Source: CAD feature listing. Evaluate the final solid. Frame: model axes, mm. Face numbers are marked on the shaded views. A direction names the side the tool comes from. Give positions to 0.01 mm unless a question says otherwise; leave off trailing zeros. Write each loop counter-clockwise with the first axis right and the second up, starting at its lowest first coordinate (ties: lowest second). Pieces come first, ordered by that corner, then holes. Notation, with made-up numbers: (56, 59.25) -> (101, 59.25) arc R27 cw to (101, 79.25) -> close; hole circle Ø3 at (85, 56.25). An arc over 180 degrees is marked (long way). Use one line per item in the form item = value. Start each with the question number.
(1) Draft query along X for the marked faces 1, 2 and 3. Return one class per face: pulls with the +X half, pulls with the -X half, needs draft (parallel to the pull), parting line crosses it, or undercut.
(2) First-contact query: P1, Ø2.5, axis at x = 47, y = 22.5, coming from the -Z side; P2, Ø12, axis at x = 46.5, z = 16.5, coming from the +Y side; P3, Ø6.5, axis at y = 37, z = 72, coming from the -X side. Flat tips, straight axial feed; report the tip coordinate or a pass-through.
(3) Material intervals for line 1 along Y through (x, z) = (45.6, 72.9); line 2 along Y through (x, z) = (48.9, 72.9); line 3 along X through (y, z) = (25.5, 75.5), sorted ascending. Write a range as from..to.
(4) Cut plane B-B, the plane y = 32. Output: boundary loops of the cut face in (x, z).
(5) Set-up query: the marked faces 4, 5 and 6. Return all of +Z, -Z, +X, -X, +Y, -Y with unobstructed straight access to the full face (end or side cutting, diameter ignored); none if empty.
(6) Cut plane A-A, the plane z = 56. Output: boundary loops of the cut face in (x, y).
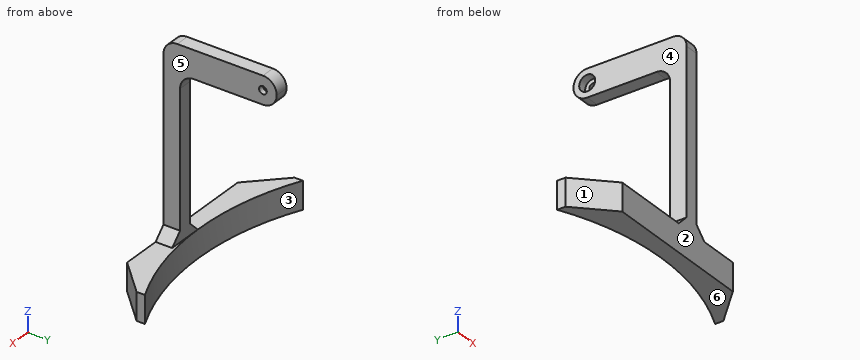
Autodesk Inventor part; units mm, degrees
ref_plane "YZ Plane" through (0, 0, 0) normal (1, 0, 0) x (0, 1, 0)
ref_plane "XZ Plane" through (0, 0, 0) normal (0, 1, 0) x (-1, 0, 0)
ref_plane "XY Plane" through (0, 0, 0) normal (0, 0, 1) x (1, 0, 0)
sketch "Esquisse1" plane through (0, 0, 0) normal (0, 0, 1) x (1, 0, 0)
  line L0 (0, 0) -> (0, 15)
  line L1 (0, 0) -> (80, 0)
  line L2 (80, 0) -> (80, 15)
  arc A0 (0, 15) -> (80, 15) centre (40, 99.3889) ccw
  line L3 (0, 6) -> (80, 6) construction
  line L4 (40, 0) -> (40, 6) construction
  dimension "d0" = 15
  dimension "d1" = 80
  dimension "d28" = 6
extrude "Extrusion1" add sketch "Esquisse1" along normal blind 10
sketch "Esquisse2" plane through (0, 0, 10) normal (0, 0, 1) x (1, 0, 0)
  line L0 (0, 0) -> (80, 0)
  line L1 (44.6, 0) -> (49.6, 0)
  line L2 (49.6, 0) -> (49.6, 6)
  line L3 (49.6, 6) -> (44.6, 6)
  line L4 (44.6, 6) -> (44.6, 0)
  line L5 (0, 15) -> (0, 0)
  line L6 (0, 6) -> (80, 6) construction
  line L7 (80, 0) -> (80, 15)
  arc A0 (0, 15) -> (80, 15) centre (40, 99.3889) ccw
  line L8 (40, 0) -> (40, 6) construction
  dimension "d6" = 5
  dimension "d9" = 80
  dimension "d11" = 6
  dimension "d27" = 4.6
extrude "Extrusion2" add sketch "Esquisse2" along normal blind 67.9 contours L4 L3 L2 L0
sketch "Esquisse6" plane through (44.6, 6, 10) normal (0, 1, 0) x (1, 0, 0)
  line L0 (5, 0) -> (5, -67.9)
  line L1 (0, 0) -> (0, -67.9)
  line L2 (5, -67.9) -> (0, -67.9)
  line L3 (0, -67.9) -> (0, -57.9)
  line L4 (0, -57.9) -> (5, -57.9)
  line L5 (5, -57.9) -> (5, -67.9)
  point P0 (-44.6, 10)
  point P1 (5, -57.9)
  dimension "d29" = 10
extrude "Extrusion5" add sketch "Esquisse6" along normal blind 35
sketch "Esquisse7" plane through (44.6, 0, 10) normal (-1, 0, 0) x (0, 0, 1)
  line L0 (67.9, 41) -> (57.9, 41) construction
  line L1 (62.9, 41) -> (62.9, 0) construction
  line L2 (0, 0) -> (67.9, 0) construction
  circle A0 centre (62.9, 36) radius 2.9
  circle A1 centre (62.9, 36) radius 1.4
  point P0 (-10, 0)
  dimension "d38" = 2.8
  dimension "d53" = 5.8
  dimension "d54" = 5
extrude "Extrusion6" cut sketch "Esquisse7" against normal up to surface (5 mm away) contours A1
chamfer "Chanfrein1" distance 4 angle 45 2 edges at (44.6, 3, 10) (49.6, 3, 10)
fillet "Congé1" radius 5 2 edges at (47.1, 0, 77.9) (47.1, 6, 67.9)
fillet "Congé2" radius 5 2 edges at (47.1, 41, 77.9) (47.1, 41, 67.9)
chamfer "Chanfrein2" distance 12 angle 45 2 edges at (0, 0, 5) (80, 0, 5)
extrude "Extrusion8" cut sketch "Esquisse7" against normal blind 3
properties part number "_Impression 3D"
Geometry says:
q1.face_1 = pulls with the -X half
q1.face_2 = needs draft
q1.face_3 = undercut
q2.P1 = 67.9
q2.P2 = 6
q2.P3 = 44.6
q3.line_1 = 0..33.1, 38.9..41
q3.line_2 = 0..34.6, 37.4..41
q3.line_3 = 44.6..49.6
q4.outline = (44.6, 67.9) -> (49.6, 67.9) -> (49.6, 77.9) -> (44.6, 77.9) -> close
q5.face_4 = +Z, -X, +Y, -Y
q5.face_5 = +Z, +X, +Y, -Y
q5.face_6 = -Z, +X, -X, +Y, -Y
q6.outline = (44.6, 0) -> (49.6, 0) -> (49.6, 6) -> (44.6, 6) -> close
